The model under review builds one solid part; all positions refer to its coordinate system, in mm. A direction names the side the tool comes from. Coordinates: 2 decimals unless noted, no trailing zeros. Order: outer loops, then holes, each group sorted by start corner. A loop starts at its lowest first (then second) coordinate and runs counter-clockwise, first axis right, second up.
```python
from build123d import *

# Parameters (mm, degrees)
SKETCH1_R           = 2.413
SKETCH1_R_2         = 0.75
BOSS_EXTRUDE1_DEPTH = 2


with BuildPart() as part:
    # Sketch1 → Boss-Extrude1 (new, symmetric)
    with BuildSketch(Plane(origin=(0, 0, 0), x_dir=(0, 0, -1), z_dir=(1, 0, 0))):
        Polygon((-43.032150888, 7.041925615), (7.041925615, 7.041925615), (7.041925615, -59.627321198), (-7.041925615, -59.627321198), (-7.041925615, -7.041925615), (-43.032150888, -7.041925615), align=None)
        Circle(SKETCH1_R, mode=Mode.SUBTRACT)
        with Locations((-5.791925615, -54.627321198)):
            Circle(SKETCH1_R_2, mode=Mode.SUBTRACT)
        with Locations((-3.64647107, -54.627321198)):
            Circle(SKETCH1_R_2, mode=Mode.SUBTRACT)
        with Locations((-1.501016524, -54.627321198)):
            Circle(SKETCH1_R_2, mode=Mode.SUBTRACT)
        with Locations((0.644438021, -54.627321198)):
            Circle(SKETCH1_R_2, mode=Mode.SUBTRACT)
        with Locations((2.789892567, -54.627321198)):
            Circle(SKETCH1_R_2, mode=Mode.SUBTRACT)
        with Locations((4.935347112, -54.627321198)):
            Circle(SKETCH1_R_2, mode=Mode.SUBTRACT)
    extrude(amount=BOSS_EXTRUDE1_DEPTH, both=True)


solid = part.part
```
(1) For pin 1 Ø0.9 at (y, z) = (-54.63, -4.94) entering from -X; pin 2 Ø2 at (x, z) = (0, 9.5) entering from -Y; pin 3 Ø2 at (x, y) = (1.5, -30) entering from +Z, all flat-tipped, find the tip position at first contact; note any pin that passes through.
A:
pin 1: passes through
pin 2: stops at y = -7.04
pin 3: stops at z = 7.04
(2) Machinability: for faces 5 (the face through (0, -34, 7.042)), 6 (the face through (2, -18.4, 6.5)), which of the approach directions +Z, -Z, +X, -X, +Y, -Y give a long, thin tool a straight path to every point of the face, cutting with its end or side? Answer none if there is none.
A:
face 5: +Z, +X, -X, -Y
face 6: +Z, -Z, +X, +Y, -Y
(3) We need section C-C, the plane z = 21.5. Write out the cut boundary in (x, y), and give its area (3 significant figures).
A:
outline: (-2, -7.04) - (2, -7.04) - (2, 7.04) - (-2, 7.04) - close
area: 56.3 mm2
(4) We need section A-A, the plane y = 0. Write out the cut boundary in (x, z).
A:
outline: (-2, -7.04) - (2, -7.04) - (2, -2.41) - (-2, -2.41) - close; (-2, 2.41) - (2, 2.41) - (2, 43.03) - (-2, 43.03) - close
(5) We need section B-B, the plane x = -0.2. Write out the cut boundary in (y, z).
A:
outline: (-59.63, -7.04) - (7.04, -7.04) - (7.04, 43.03) - (-7.04, 43.03) - (-7.04, 7.04) - (-59.63, 7.04) - close; hole circle Ø1.5 at (-54.63, -4.94); hole circle Ø1.5 at (-54.63, -2.79); hole circle Ø1.5 at (-54.63, -0.64); hole circle Ø1.5 at (-54.63, 1.5); hole circle Ø1.5 at (-54.63, 3.65); hole circle Ø1.5 at (-54.63, 5.79); hole circle Ø4.83 at (0, 0)
(6) Wall thickness on probe 1 along Y at (x, z) = (-0.65, 3.5); probe 2 along Z at (x, y) = (0.05, -34.5); probe 3 along Y at (x, z) = (-1.25, -3): over which ranges is each line inside the solid? List them lowest first.
A:
probe 1: y = -59.63 to -55.36, -53.89 to 7.04
probe 2: z = -7.04 to 7.04
probe 3: y = -59.63 to -55.35, -53.91 to 7.04
(7) Draft analysis for pull direction Y (two halves, no side actions). For faces 1 (the face through (-0.028, -54.402, 5.077)), 2 (the face through (0, -26, -7.042)), 3 (the face through (0, -54, -3.2)), 4 (the face through (0, -59.627, 0)), state which applies: released by +Y, released by -Y, zero draft, split by the parting line, or undercut.
A:
face 1: undercut
face 2: zero draft
face 3: undercut
face 4: released by -Y
